Input: part model. Units: mm. Frame: model coordinates. A direction names the side the tool comes from. Coordinates: 2 decimals unless noted, no trailing zeros. Order: outer loops, then holes, each group sorted by start corner. A loop starts at its lowest first (then second) coordinate and runs counter-clockwise, first axis right, second up. Notation, with made-up numbers: (76, 41.5) -> (133, 41.5) arc R15 cw to (133, 55.5) -> close; hole circle Ø2 at (66.25, 73). An arc over 180 degrees is marked (long way). Use one line per item in the form item = value. Start each with the question number.
1) Pin query (flat end, axial travel): pin 1 (1 mm diameter, centred on x = 4, z = 2, fed in from +Y); pin 2 (0.7 mm diameter, centred on x = 0.5, z = -1.5, fed in from +Y); pin 3 (0.7 mm diameter, centred on x = 0.5, y = 0, fed in from -Z). Return the tip coordinate at first contact, or that it passes through.
2) Section query B-B on x = 2.6. Output: boundary loops of the cut face in (y, z).
3) Section query A-A on y = 0. Output: boundary loops of the cut face in (x, z), then the cut area to 3 significant figures.
4) Section query C-C on x = 1.65. Output: boundary loops of the cut face in (y, z).
5) Draft query along Y for faces 4 (the flat face through (0.5, -0.467, 1.3)), 5 (the conical face through (1.875, -0.279, -2.123)), 6 (the flat face through (5, 0, 0)), 7 (the flat face through (0.5, 1.75, 0)). Return one class per face: pulls with the +Y half, pulls with the -Y half, needs draft (parallel to the pull), parting line crosses it, or undercut.
6) Access query for faces 1 (the flat face through (0, 1, -1)), 2 (the cylindrical face through (3, 0, -2)), 3 (the flat face through (0.5, 1.3, -0.467)). Directions: +Z, -Z, +X, -X, +Y, -Y. A direction counts if a zero-diameter tool reaches every point of the face in a straight line with its end or side. Return the directions, or none.
7) Ray query, line 1 along X through (y, z) = (0, 1.5); line 2 along X through (y, z) = (-1.75, 3.25); line 3 along Y through (x, z) = (3, 1.5). Return the intervals inside material, ascending.
Autodesk Inventor part; units mm, degrees
ref_plane "screw_XY" through (2, 0, 0) normal (1, 0, 0) x (0, 0, -1)
ref_plane "screw_YZ" through (2, 0, 0) normal (0, 0, -1) x (0, 1, 0)
ref_plane "screw_ZX" through (2, 0, 0) normal (0, 1, 0) x (1, 0, 0)
sketch "Sketch_1" plane through (0, 0, 0) normal (0, 0, 1) x (1, 0, 0)
  line L0 (5, 0) -> (0, 0)
  line L1 (0, 0) -> (0, 4.25)
  line L2 (0, 4.25) -> (2, 2)
  line L3 (2, 2) -> (4.5705, 2)
  line L4 (4.5705, 2) -> (5, 1.5705)
  line L5 (5, 1.5705) -> (5, 0)
  line L6 (5, 0) -> (0, 0)
revolve "Revolution1" add sketch "Sketch_1" angle 360 about axis through (5, 0, 0) along (1, 0, 0)
thread "Thread1"
sketch "_____1" plane through (0, 0, 0) normal (1, 0, 0) x (0, 0, -1)
  line L0 (-1.75, 0.4667) -> (-1.75, -0.4667)
  line L1 (-1.75, -0.4667) -> (-0.9333, -0.4667)
  arc A0 (-0.4667, -0.9333) -> (-0.9333, -0.4667) centre (-0.9333, -0.9333) ccw
  line L2 (-0.4667, -0.9333) -> (-0.4667, -1.75)
  line L3 (-0.4667, -1.75) -> (0.4667, -1.75)
  line L4 (0.4667, -1.75) -> (0.4667, -0.9333)
  arc A1 (0.9333, -0.4667) -> (0.4667, -0.9333) centre (0.9333, -0.9333) ccw
  line L5 (0.9333, -0.4667) -> (1.75, -0.4667)
  line L6 (1.75, -0.4667) -> (1.75, 0.4667)
  line L7 (1.75, 0.4667) -> (0.9333, 0.4667)
  arc A2 (0.4667, 0.9333) -> (0.9333, 0.4667) centre (0.9333, 0.9333) ccw
  line L8 (0.4667, 0.9333) -> (0.4667, 1.75)
  line L9 (0.4667, 1.75) -> (-0.4667, 1.75)
  line L10 (-0.4667, 1.75) -> (-0.4667, 0.9333)
  arc A3 (-0.9333, 0.4667) -> (-0.4667, 0.9333) centre (-0.9333, 0.9333) ccw
  line L11 (-0.9333, 0.4667) -> (-1.75, 0.4667)
extrude "Extrusion1" cut sketch "_____1" along normal blind 1
ref_plane "screw_XY" through (2, 0, 0) normal (1, 0, 0) x (0, 0, -1)
ref_plane "screw_YZ" through (2, 0, 0) normal (0, 0, -1) x (0, 1, 0)
ref_plane "screw_ZX" through (2, 0, 0) normal (0, 1, 0) x (1, 0, 0)
properties part number "FBb4-5"
Answers below:
q1.pin_1 = 1.32
q1.pin_2 = 3.82
q1.pin_3 = -4.08
q2.outline = circle Ø4 at (0, 0)
q3.outline = (0, -4.25) -> (2, -2) -> (4.57, -2) -> (5, -1.57) -> (5, 1.57) -> (4.57, 2) -> (2, 2) -> (0, 4.25) -> (0, 1.75) -> (1, 1.75) -> (1, -1.75) -> (0, -1.75) -> close
q3.area = 20.8 mm^2
q4.outline = circle Ø4.79 at (0, 0)
q5.face_4 = undercut
q5.face_5 = parting line crosses it
q5.face_6 = needs draft
q5.face_7 = undercut
q6.face_1 = +Z, -Z, -X, +Y, -Y
q6.face_2 = +X
q6.face_3 = -X
q7.line_1 = 1 to 5
q7.line_2 = 0 to 0.5
q7.line_3 = -1.32 to 1.32
